For this review, use the dimensioned drawing (mm, ordinates from the lowest corner) and the shaded views. A direction names the side the tool comes from. Give positions to 0.01 mm unless a question says otherwise; leave off trailing zeros. Order: outer loops, then holes, each group sorted by start corner. A loop starts at its lowest first (then second) coordinate and runs counter-clockwise, first axis right, second up. Notation, with made-up numbers: (-16.75, 84.5) - (23.25, 84.5) arc R36 cw to (23.25, 119.5) - close; hole circle Ø1 at (34.25, 42). An arc over 180 degrees is marked (long way). Use a Markdown table: item, result. Add a question column.
1) Clearance check with flat-ended pins moving along their axes: P1, Ø5, axis at x = 13, y = 8.5, coming from the -Z side; P2, Ø1, axis at y = 3.5, z = 13.5, coming from the +X side; P3, Ø2, axis at x = 11.5, z = 6.5, coming from the -Y side. State where each tip first meets the part, or that it passes through.
2) Wall thickness on L1, parallel to X at y = 3.75, z = 15.25; L2, parallel to X at y = 4.75, z = 12; L3, parallel to Y at x = 66.5, z = 18.5: over which ranges is each line inside the solid? List them lowest first.
3) Machinability: for the marked faces 1 and 2, which of the approach directions +Z, -Z, +X, -X, +Y, -Y give a long, thin tool a straight path to every point of the face, cutting with its end or side? Answer none if there is none.
4) We need section D-D on x = 54. Write out the cut boundary in (y, z), then the cut area to 3 significant figures.
5) We need section C-C on y = 6.25. Write out the cut boundary in (x, z).
6) We need section A-A on z = 15. Write out the cut boundary in (x, y), then the cut area to 3 significant figures.
7) We need section B-B on x = 69. Write out the cut boundary in (y, z).
8) Mouldability with a two-part tool opening along X and no side actions: class the marked faces 3 and 4 as released by +X, released by -X, zero draft, split by the parting line, or undercut.
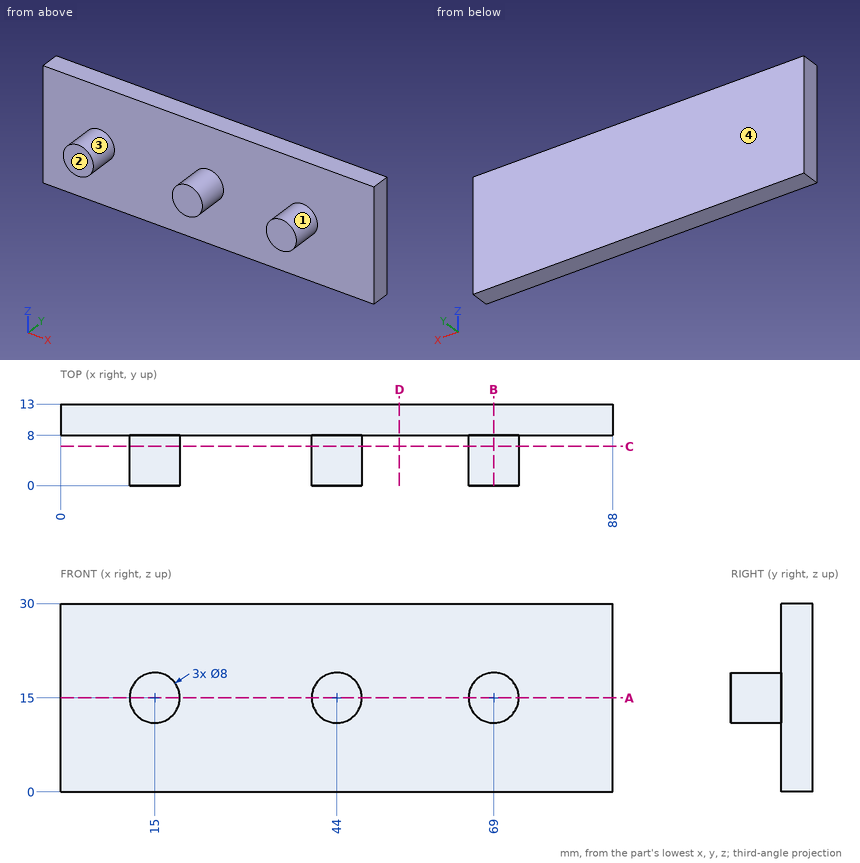
Checked values:
| question | item | result |
|---|---|---|
| 1 | P1 | z = 0 |
| 1 | P2 | x = 72.87 |
| 1 | P3 | y = 8 |
| 2 | L1 | 11.01 to 18.99, 40.01 to 47.99, 65.01 to 72.99 |
| 2 | L2 | 12.35 to 17.65, 41.35 to 46.65, 66.35 to 71.65 |
| 2 | L3 | 8 to 13 |
| 3 | face 1 | -Y |
| 3 | face 2 | +Z, -Z, +X, -X, -Y |
| 4 | outline | (8, 0) - (13, 0) - (13, 30) - (8, 30) - close |
| 4 | area | 150 mm² |
| 5 | outline | circle Ø8 at (15, 15); circle Ø8 at (44, 15); circle Ø8 at (69, 15) |
| 6 | outline | (0, 8) - (11, 8) - (11, 0) - (19, 0) - (19, 8) - (40, 8) - (40, 0) - (48, 0) - (48, 8) - (65, 8) - (65, 0) - (73, 0) - (73, 8) - (88, 8) - (88, 13) - (0, 13) - close |
| 6 | area | 632 mm² |
| 7 | outline | (0, 11) - (8, 11) - (8, 0) - (13, 0) - (13, 30) - (8, 30) - (8, 19) - (0, 19) - close |
| 8 | face 3 | undercut |
| 8 | face 4 | zero draft |
